Source: CAD feature listing. Evaluate the final solid. Frame: model axes, mm. Face numbers are marked on the shaded views. A direction names the side the tool comes from. Give positions to 0.01 mm unless a question says otherwise; leave off trailing zeros. Loops run counter-clockwise (first coordinate to the right, second up) from the corner with the lowest first, then second, coordinate; pieces in that order, holes last. Notation, with made-up numbers: (13, 84) -> (71, 84) arc R11 ccw to (71, 103) -> close; hole circle Ø5 at (-25.75, -20.5). An arc over 180 degrees is marked (long way). Return JSON: item names as keys, results as strings. Group by question number.
```python
from build123d import *

# Parameters (mm, degrees)
DODANIE_WYCI_GNI_CIE1_DEPTH = 5
SZKIC2_W                    = 75
SZKIC2_H                    = 35
DODANIE_WYCI_GNI_CIE2_DEPTH = 5
SZKIC3_R                    = 6
WYTNIJ_WYCI_GNI_CIE1_DEPTH  = 86.586213843


with BuildPart() as part:
    # Szkic1 → Dodanie-wyci_gni_cie1 (new body)
    with BuildSketch(Plane.XY):
        with BuildLine():
            Line((-50, -20), (50, -20))
            Line((50, -20), (50, 20))
            Line((50, 20), (-50, 20))
            ThreePointArc((-50, 20), (-70, 0), (-50, -20))
        make_face()
    extrude(amount=DODANIE_WYCI_GNI_CIE1_DEPTH)


with BuildPart() as body_2:
    # Lustro2: mirrored copy
    add(part.part.mirror(Plane.XY.offset(22.5)))


with BuildPart() as part_1:
    add(part.part)

    add(body_2.part)  # Dodanie-wyci_gni_cie2 merges body 2
    # Szkic2 → Dodanie-wyci_gni_cie2 (add)
    with BuildSketch(Plane(origin=(0, 20, 0), x_dir=(1, 0, 0), z_dir=(0, 1, 0))):
        with Locations((12.5, -22.5)):
            Rectangle(SZKIC2_W, SZKIC2_H)
    dodanie_wyci_gni_cie2 = extrude(amount=-DODANIE_WYCI_GNI_CIE2_DEPTH)

    # Lustro5: Dodanie-wyci_gni_cie2 across plane
    add(dodanie_wyci_gni_cie2.mirror(Plane.ZX))

    # Szkic3 → Wytnij-wyci_gni_cie1 (cut, through all)
    with BuildSketch(Plane(origin=(0, 0, 0), x_dir=(-1, 0, 0), z_dir=(0, 0, -1))):
        with Locations((50, 0)):
            Circle(SZKIC3_R)
    extrude(amount=-WYTNIJ_WYCI_GNI_CIE1_DEPTH, mode=Mode.SUBTRACT)


solid = part_1.part
```
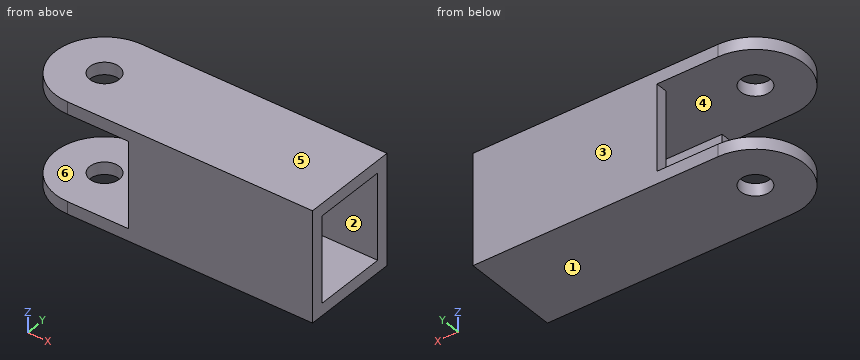
1) Cut plane D-D on y = -10.5. Return loops of the section in (x, z), then the cut area to 3 significant figures.
2) Reachability of the marked faces 1 and 2 from +Z, -Z, +X, -X, +Y, -Y: full face, straight path, thin tool, end or side. Return the list, or none.
3) Cut plane C-C on z = 23. Return loops of the section in (x, y).
4) Material intervals for line 1 (Z direction, x = -10, y = 1.5); line 2 (Y direction, x = -22, z = 10); line 3 (Y direction, x = -50, z = 41), sorted ascending.
5) Cut plane A-A on x = 8. Return loops of the section in (y, z).
6) Contact query for flat-ended pins moving along their axis: P1, Ø1.5, axis at y = -18.5, z = 26.5, coming from the -X side; P2, Ø20, axis at x = -30.5, y = -4.5, coming from the -Z side. Output: stop coordinate, or through.
7) Cut plane B-B on y = 0. Return loops of the section in (x, z).
8) Mould query, pull axis Y, two halves, no side actions, for the marked faces 3, 4, 5 and 6. Classes: released by +Y, released by -Y, zero draft, split by the parting line, or undercut.
Calculated:
{
 "1": {"outline": "(-67.02, 0) -> (50, 0) -> (50, 5) -> (-67.02, 5) -> close; (-67.02, 40) -> (50, 40) -> (50, 45) -> (-67.02, 45) -> close", "area": "1,170 mm2"},
 "2": {"face 1": "-Z, +X, -X, +Y, -Y", "face 2": "+X, -X"},
 "3": {"outline": "(-25, -20) -> (50, -20) -> (50, -15) -> (-25, -15) -> close; (-25, 15) -> (50, 15) -> (50, 20) -> (-25, 20) -> close"},
 "4": {"line 1": "0 to 5, 40 to 45", "line 2": "-20 to -15, 15 to 20", "line 3": "-20 to -6, 6 to 20"},
 "5": {"outline": "(-20, 0) -> (20, 0) -> (20, 45) -> (-20, 45) -> close; hole (-15, 5) -> (15, 5) -> (15, 40) -> (-15, 40) -> close"},
 "6": {"P1": "x = -25", "P2": "z = 0"},
 "7": {"outline": "(-70, 0) -> (-56, 0) -> (-56, 5) -> (-70, 5) -> close; (-70, 40) -> (-56, 40) -> (-56, 45) -> (-70, 45) -> close; (-44, 0) -> (50, 0) -> (50, 5) -> (-44, 5) -> close; (-44, 40) -> (50, 40) -> (50, 45) -> (-44, 45) -> close"},
 "8": {"face 3": "released by +Y", "face 4": "undercut", "face 5": "zero draft", "face 6": "undercut"}
}
